from build123d import *

# Parameters (mm, degrees)
EXTRUDE_1_DEPTH = 1
FILLET_1_R      = 1.5


with BuildPart() as part:
    # 草图1 → 凸台-拉伸1 (new body)
    with BuildSketch(Plane(origin=(0, 0, 0), x_dir=(1, 0, 0), z_dir=(0, 1, 0))):
        Polygon((-24.804006769, -20.720140696), (-4.804006769, -20.720140696), (-4.804006769, -0.720140696), (-12.304006769, -0.720140696), (-12.304006769, 29.279859304), (-17.304006769, 29.279859304), (-17.304006769, -0.720140696), (-24.804006769, -0.720140696), align=None)
    extrude(amount=EXTRUDE_1_DEPTH)

    # 圆角1
    fillet_1_edges = [part.edges().sort_by_distance(p)[0] for p in [
        (-24.804006769, 0.5, 0.720140696),
        (-17.304006769, 0.5, -29.279859304),
        (-12.304006769, 0.5, -29.279859304),
        (-4.804006769, 0.5, 0.720140696),
        (-4.804006769, 0.5, 20.720140696),
        (-24.804006769, 0.5, 20.720140696),
    ]]
    fillet(fillet_1_edges, radius=FILLET_1_R)


solid = part.part
Could you check a few things on this model? Use its own coordinates, in mm. A direction names the side the tool comes from. Give positions to 0.01 mm unless a question says otherwise; leave off trailing zeros. Loops run counter-clockwise (first coordinate to the right, second up) from the corner with the lowest first, then second, coordinate; pieces in that order, holes last. Notation, with made-up numbers: M 9,43 L 38,43 A9 ccw 38,58 Z; hole C -8,13.25 d1. An arc over 180 degrees is marked long. Answer as a JSON object with one key per item and string values.
Q1. For P1, Ø0.5, axis at y = 0.5, z = -17, coming from the -X side, with a flat end and sliding along its axis, tell me the tip position at first contact or that it passes through.
Values found:
{"P1": "stops at x = -17.3"}
Q2. Suppose I cut it at C-C, the plane z = -23. List the corners of the cut face in (x, y) for me.
Values found:
{"outline": "M -17.3,0 L -12.3,0 L -12.3,1 L -17.3,1 Z"}
Q3. If I drill on probe 1 along X at (y, z) = (0.45, -19.5); probe 2 along Z at (x, y) = (-10, 0.7); probe 3 along Z at (x, y) = (-6, 0.9), over which ranges is the centre line in solid material (lowest first)? Write a range as [from, to].
Values found:
{"probe 1": "x = [-17.3, -12.3]", "probe 2": "z = [0.72, 20.72]", "probe 3": "z = [0.75, 20.69]"}
Q4. For faces 1 (the flat face through (-9.3, 0.5, 0.72)), 2 (the flat face through (-17.304, 0.5, -13.7)), 3 (the cylindrical face through (-24.353, 0.507, 20.292)), which set-ups out of +Z, -Z, +X, -X, +Y, -Y let a thin tool reach every point of the face, with its end or its side?
Values found:
{"face 1": "-Z, +X, +Y, -Y", "face 2": "-Z, -X, +Y, -Y", "face 3": "+Z, -X, +Y, -Y"}
Q5. Suppose I cut it at B-B, the plane x = -6.75. List the corners of the cut face in (y, z) for me.
Values found:
{"outline": "M 0,0.72 L 1,0.72 L 1,20.72 L 0,20.72 Z"}
Q6. Suppose I cut it at A-A, the plane y = 0.4. List the corners of the cut face in (x, z) for me, plus the area to 3 significant figures.
Values found:
{"outline": "M -24.8,2.22 A1.5 ccw -23.3,0.72 L -17.3,0.72 L -17.3,-27.78 A1.5 ccw -15.8,-29.28 L -13.8,-29.28 A1.5 ccw -12.3,-27.78 L -12.3,0.72 L -6.3,0.72 A1.5 ccw -4.8,2.22 L -4.8,19.22 A1.5 ccw -6.3,20.72 L -23.3,20.72 A1.5 ccw -24.8,19.22 Z", "area": "547 mm²"}
